CAD build for the part. Positions are in the model's coordinates, mm. A direction names the side the tool comes from. Give positions to 0.01 mm unless a question says otherwise; leave off trailing zeros. Order: outer loops, then holes, each group sorted by start corner. A loop starts at its lowest first (then second) coordinate and runs counter-clockwise, first axis right, second up. Notation, with made-up numbers: (62, 45) -> (83, 45) arc R22 ccw to (83, 63) -> close; hole circle Ø10 at (44, 86). An arc over 180 degrees is marked (long way). Answer as CSV lines item,"result".
```python
from build123d import *

# Parameters (mm, degrees)
F0_R         = 5.7
F1_DEPTH     = 70
F2_R         = 5.7
F3_DEPTH     = 5
F5_DEPTH     = 5
F6_W         = 5.4
F6_H         = 3.5
F7_DEPTH     = 2.7
F8_R         = 2.5
F9_T4_ANGLE  = 295.1748403761
F9_T9_ANGLE  = 295.1748403761
F9_T15_ANGLE = 295.1748403761
F9_T20_ANGLE = 295.1748403761
F9_T25_ANGLE = 295.1748403761
F9_T31_ANGLE = 295.1748403761


# Not quite as in the source:
# - a fillet or chamfer that OpenCascade refuses, or shapes differently, is made with other operations: its cross-section is extruded or revolved along the edge and cut away or added


with BuildPart() as f1:
    # F0 (on Top) → F1 (new body)
    with BuildSketch(Plane.XY):
        Circle(F0_R)
        Polygon((-2.136195996, -3.7), (-4.272391992, 0), (-2.136195996, 3.7), (2.136195996, 3.7), (4.272391992, 0), (2.136195996, -3.7), align=None, mode=Mode.SUBTRACT)
    extrude(amount=F1_DEPTH)

    # F2 (on face) → F3 (join)
    with BuildSketch(Plane.XY.offset(70)):
        Circle(F2_R)
        Polygon((2.136195996, -3.7), (-2.136195996, -3.7), (-4.272391992, 0), (-2.136195996, 3.7), (2.136195996, 3.7), (4.272391992, 0), align=None, mode=Mode.SUBTRACT)
        Polygon((-4.272391992, 0), (-2.136195996, -3.7), (2.136195996, -3.7), (4.272391992, 0), (2.136195996, 3.7), (-2.136195996, 3.7), align=None)
    extrude(amount=F3_DEPTH)

    # F4 (on face) → F5 (join)
    with BuildSketch(Plane.XY.offset(75)):
        with BuildLine():
            Line((-5.4247119739, -1.75), (-2.7, -1.75))
            Line((-2.7, -1.75), (-2.7, 1.75))
            Line((-2.7, 1.75), (-5.4247119739, 1.75))
            ThreePointArc((-5.4247119739, 1.75), (-5.7, 0), (-5.4247119739, -1.75))
        make_face()
        with BuildLine():
            Line((2.7, -1.75), (5.4247119739, -1.75))
            ThreePointArc((5.4247119739, -1.75), (5.6307574202, -0.8857600546), (5.7, 0))
            ThreePointArc((5.7, 0), (5.6307574202, 0.8857600546), (5.4247119739, 1.75))
            Line((5.4247119739, 1.75), (2.7, 1.75))
            Line((2.7, 1.75), (2.7, -1.75))
        make_face()
    extrude(amount=F5_DEPTH)

    # F6 (on face) → F7 (join)
    with BuildSketch(Plane.XY.offset(80)):
        Rectangle(F6_W, F6_H)
        with BuildLine():
            Line((-2.7, -1.75), (-2.7, 1.75))
            Line((-2.7, 1.75), (-5.4247119739, 1.75))
            ThreePointArc((-5.4247119739, 1.75), (-5.7, 0), (-5.4247119739, -1.75))
            Line((-5.4247119739, -1.75), (-2.7, -1.75))
        make_face()
        with BuildLine():
            Line((5.4247119739, 1.75), (2.7, 1.75))
            Line((2.7, 1.75), (2.7, -1.75))
            Line((2.7, -1.75), (5.4247119739, -1.75))
            ThreePointArc((5.4247119739, -1.75), (5.7, 0), (5.4247119739, 1.75))
        make_face()
    extrude(amount=F7_DEPTH)

    # F8
    f8_edges = [f1.edges().sort_by_distance(p)[0] for p in [
        (-5.7, 0, 82.7),
        (2.7, 0, 80),
        (-2.7, 0, 80),
        (5.7, 0, 82.7),
    ]]
    fillet(f8_edges, radius=F8_R)

    # F9: fillet of radius 3 on 3 edges, made by hand


with BuildPart() as f9_tool2:
    # F9_s3 → F9_t4 (revolve)
    with BuildSketch(Plane(origin=(0, 0, 0), x_dir=(0, 0, 1), z_dir=(0.8442102595, 0.536012162, 0))):
        with BuildLine():
            ThreePointArc((72, -5.7), (74.1213203436, -4.8213203436), (75, -2.7))
            Line((75, -2.7), (75, -5.7))
            Line((75, -5.7), (72, -5.7))
        make_face()
    revolve(axis=Axis((0, 0, 75), (0, 0, 1)), revolution_arc=F9_T4_ANGLE)

    split(bisect_by=Plane.XZ.offset(-1.75), keep=Keep.BOTTOM)


with BuildPart() as f1_1:
    add(f1.part)

    # F9_t1: cut F9_tool2
    add(f9_tool2.part, mode=Mode.SUBTRACT)


with BuildPart() as f9_tool7:
    # F9_s8 → F9_t9 (revolve)
    with BuildSketch(Plane(origin=(0, 0, 0), x_dir=(0, 0, 1), z_dir=(0.8442102595, 0.536012162, 0))):
        with BuildLine():
            ThreePointArc((72, -5.7), (74.1213203436, -4.8213203436), (75, -2.7))
            Line((75, -2.7), (75, -5.7))
            Line((75, -5.7), (72, -5.7))
        make_face()
    revolve(axis=Axis((0, 0, 75), (0, 0, 1)), revolution_arc=F9_T9_ANGLE)

    split(bisect_by=Plane.YZ.offset(-2.7), keep=Keep.TOP)

    split(bisect_by=Plane.YZ.offset(2.7), keep=Keep.BOTTOM)


with BuildPart() as f1_2:
    add(f1_1.part)

    # F9_t6: cut F9_tool7
    add(f9_tool7.part, mode=Mode.SUBTRACT)


with BuildPart() as f9_tool13:
    # F9_s14 → F9_t15 (revolve)
    with BuildSketch(Plane(origin=(0, 0, 0), x_dir=(0, 0, 1), z_dir=(0.8442102595, 0.536012162, 0))):
        with BuildLine():
            ThreePointArc((72, -5.7), (74.1213203436, -4.8213203436), (75, -2.7))
            Line((75, -2.7), (75, -5.7))
            Line((75, -5.7), (72, -5.7))
        make_face()
    revolve(axis=Axis((0, 0, 75), (0, 0, 1)), revolution_arc=F9_T15_ANGLE)

    split(bisect_by=Plane.XZ.offset(1.75), keep=Keep.TOP)


with BuildPart() as f1_3:
    add(f1_2.part)

    # F9_t12: cut F9_tool13
    add(f9_tool13.part, mode=Mode.SUBTRACT)


with BuildPart() as f9_tool18:
    # F9_s19 → F9_t20 (revolve)
    with BuildSketch(Plane(origin=(0, 0, 0), x_dir=(0, 0, 1), z_dir=(-0.8442102595, -0.536012162, 0))):
        with BuildLine():
            ThreePointArc((72, -5.7), (74.1213203436, -4.8213203436), (75, -2.7))
            Line((75, -2.7), (75, -5.7))
            Line((75, -5.7), (72, -5.7))
        make_face()
    revolve(axis=Axis((0, 0, 75), (0, 0, 1)), revolution_arc=F9_T20_ANGLE)

    split(bisect_by=Plane.XZ.offset(1.75), keep=Keep.TOP)


with BuildPart() as f1_4:
    add(f1_3.part)

    # F9_t17: cut F9_tool18
    add(f9_tool18.part, mode=Mode.SUBTRACT)


with BuildPart() as f9_tool23:
    # F9_s24 → F9_t25 (revolve)
    with BuildSketch(Plane(origin=(0, 0, 0), x_dir=(0, 0, 1), z_dir=(-0.8442102595, -0.536012162, 0))):
        with BuildLine():
            ThreePointArc((72, -5.7), (74.1213203436, -4.8213203436), (75, -2.7))
            Line((75, -2.7), (75, -5.7))
            Line((75, -5.7), (72, -5.7))
        make_face()
    revolve(axis=Axis((0, 0, 75), (0, 0, 1)), revolution_arc=F9_T25_ANGLE)

    split(bisect_by=Plane.YZ.offset(-2.7), keep=Keep.TOP)

    split(bisect_by=Plane.YZ.offset(2.7), keep=Keep.BOTTOM)


with BuildPart() as f1_5:
    add(f1_4.part)

    # F9_t22: cut F9_tool23
    add(f9_tool23.part, mode=Mode.SUBTRACT)


with BuildPart() as f9_tool29:
    # F9_s30 → F9_t31 (revolve)
    with BuildSketch(Plane(origin=(0, 0, 0), x_dir=(0, 0, 1), z_dir=(-0.8442102595, -0.536012162, 0))):
        with BuildLine():
            ThreePointArc((72, -5.7), (74.1213203436, -4.8213203436), (75, -2.7))
            Line((75, -2.7), (75, -5.7))
            Line((75, -5.7), (72, -5.7))
        make_face()
    revolve(axis=Axis((0, 0, 75), (0, 0, 1)), revolution_arc=F9_T31_ANGLE)

    split(bisect_by=Plane.XZ.offset(-1.75), keep=Keep.BOTTOM)


with BuildPart() as f1_6:
    add(f1_5.part)

    # F9_t28: cut F9_tool29
    add(f9_tool29.part, mode=Mode.SUBTRACT)


solid = f1_6.part
```
1) Which spindle directions (+Z, -Z, +X, -X, +Y, -Y) get a long thin tool onto all of the face, cutting with end or side? Do faces 4 (the flat face through (0, 3.7, 35)), 5 (the flat face through (0, 0, 82.7)), 6 (the cylindrical face through (1.948, -0.025, 79.287)). Say none if no direction does.
Data:
face 4,"-Z"
face 5,"+Z, +X, -X, +Y, -Y"
face 6,"+Y, -Y"
2) Pin check, flat tips, straight feed: P1, Ø1.5, axis at x = 4, y = 4, coming from the -Z side; P2, Ø1.5, axis at x = 0, y = 1, coming from the -Z side; P3, Ø1.5, axis at y = -2.5, z = 10, coming from the -X side; P4, Ø1.3, axis at x = 1, z = 30.5, coming from the +Y side. Stop position of each tip, or through.
Data:
P1,"stops at z = 0"
P2,"stops at z = 70"
P3,"stops at x = -5.42"
P4,"stops at y = 5.69"
3) Wall check: line 1 along Y through (x, z) = (1.75, 40); line 2 along Y through (x, z) = (0, 39); line 3 along X through (y, z) = (2.25, 50.5). Give the ranges that are in metal, low to high. Write a range as [from, to].
Data:
line 1,"y = [-5.42, -3.7], [3.7, 5.42]"
line 2,"y = [-5.7, -3.7], [3.7, 5.7]"
line 3,"x = [-5.24, -2.97], [2.97, 5.24]"
4) Pull direction X, two halves, no side cores. Call faces 1 (the flat face through (3.22, -1.82, 34.51)), 2 (the flat face through (0, -3.7, 35)), 3 (the flat face through (0, 1.75, 81)): pulls with the +X half, pulls with the -X half, needs draft (parallel to the pull), parting line crosses it, or undercut.
Data:
face 1,"undercut"
face 2,"undercut"
face 3,"needs draft"
5) Band-saw the part on A-A, the plane z = 25. Write the cut outline in (x, y).
Data:
outline,"circle Ø11.4 at (0, 0); hole (-4.27, 0) -> (-2.14, -3.7) -> (2.14, -3.7) -> (4.27, 0) -> (2.14, 3.7) -> (-2.14, 3.7) -> close"
